Geometry: final body of the model. Coordinates: model frame, mm. A direction names the side the tool comes from. Round coordinates to 2 decimals unless told otherwise and drop trailing zeros. Write each loop counter-clockwise with the first axis right and the second up, starting at its lowest first coordinate (ties: lowest second). Pieces come first, ordered by that corner, then holes. Notation, with made-up numbers: (29.25, 31.5) -> (73.25, 31.5) arc R17 cw to (73.25, 57.5) -> close; hole circle Ø5 at (75.5, 72.25). An arc over 180 degrees is marked (long way). One line per item, written item: value. Start each with the question number.
from build123d import *

# Parameters (mm, degrees)
SKETCH1_R               = 10
BOSS_EXTRUDE1_DEPTH     = 35
SKETCH2_R               = 2.9
CUT_EXTRUDE1_DEPTH      = 12
CUT_EXTRUDE1_DRAFT      = -1
CUT_EXTRUDE2_DEPTH      = 38.749172176
CUT_EXTRUDE2_DEPTH_BACK = 38.749172176
SKETCH3_R               = 3
CUT_EXTRUDE3_REACH      = 39.749
CUT_EXTRUDE3_END_RADIUS = 3
SKETCH4_R               = 2.8


with BuildPart() as part:
    # Sketch1 → Boss-Extrude1 (new body)
    with BuildSketch(Plane.XY):
        Circle(SKETCH1_R)
    extrude(amount=BOSS_EXTRUDE1_DEPTH)


with BuildPart() as cut_extrude1_tool:
    # Sketch2 → Cut-Extrude1 (with draft: the straight prism first)
    with BuildSketch(Plane(origin=(0, 0, 12), x_dir=(-1, 0, 0), z_dir=(0, 0, -1))):
        Circle(SKETCH2_R)
    extrude(amount=CUT_EXTRUDE1_DEPTH)
    # Cut-Extrude1: the draft: its side faces are tilted about the plane it starts from
    cut_extrude1_sides = [cut_extrude1_tool.faces().sort_by_distance(p)[0] for p in [
        (2.9, 0, 6),
    ]]
    draft(cut_extrude1_sides, Plane(origin=(0, 0, 12), x_dir=(-1, 0, 0), z_dir=(0, 0, -1)), CUT_EXTRUDE1_DRAFT)


with BuildPart() as part_1:
    add(part.part)

    # Cut-Extrude1: cut by cut_extrude1_tool
    add(cut_extrude1_tool.part, mode=Mode.SUBTRACT)

    # Sketch3 → Cut-Extrude2 (cut, two sides: drawn at the far end of the back side and taken through both)
    with BuildSketch(Plane(origin=(0, 0, 0), x_dir=(1, 0, 0), z_dir=(0, 1, 0)).offset(-CUT_EXTRUDE2_DEPTH_BACK)):
        with Locations(Location((0, -25, 0), (0, 0, 270))):
            Circle(SKETCH3_R)
    extrude(amount=CUT_EXTRUDE2_DEPTH + CUT_EXTRUDE2_DEPTH_BACK, mode=Mode.SUBTRACT)

    # Cut-Extrude3: up to this cylinder (the profile starts outside it)
    cut_extrude3_end = Plane(origin=(0, 0, 25), z_dir=(0, 1, 0)) * Cylinder(CUT_EXTRUDE3_END_RADIUS, 86.498, mode=Mode.PRIVATE)
    # Sketch4 → Cut-Extrude3 (cut, up to the surface)
    with BuildSketch(Plane.XY.offset(35), mode=Mode.PRIVATE) as cut_extrude3_sk1:
        Circle(SKETCH4_R)
    cut_extrude3_tool1 = extrude(cut_extrude3_sk1.sketch, amount=-CUT_EXTRUDE3_REACH, mode=Mode.PRIVATE) - cut_extrude3_end
    add(cut_extrude3_tool1.solids().sort_by_distance((0, 0, 35))[0], mode=Mode.SUBTRACT)


solid = part_1.part
(1) Section query D-D (z = 32). Output: boundary loops of the cut face in (x, y), and give its area (3 significant figures).
(2) Section query B-B (x = 0). Count the separate pieces of the cut face and the enclosed holes in it, and give its area (3 significant figures).
(3) Pull-direction query (X, two-part tool) for faces 4 (the face through (-1.386, -2.664, 6.084)), 5 (the face through (9.54, 3, 17.26)), 6 (the face through (2.1, -2.1, 35)); classes: pulls with the +X half, pulls with the -X half, needs draft (parallel to the pull), parting line crosses it, or undercut.
(4) Pin query (flat end, axial travel): pin 1 (1.5 mm diameter, centred on y = -3.5, z = 6.5, fed in from +X); pin 2 (1.7 mm diameter, centred on x = 0, y = 0, fed in from -Z); pin 3 (9 mm diameter, centred on x = 0, y = 0, fed in from +Z); pin 4 (2 mm diameter, centred on y = 6.5, z = 8.5, fed in from -X). Return the tip coordinate at first contact, or that it passes through.
(5) Section query C-C (z = 21). Output: boundary loops of the cut face in (x, y).
(6) Line query: probe 1 along Y at (x, z) = (0, 29); probe 2 along X at (y, z) = (2, 29.5); probe 3 along X at (y, z) = (-2.75, 26.5). Output: solid intervals per line, ascending.
(7) Section query A-A (y = -8). Output: boundary loops of the cut face in (x, z), and give its area (3 significant figures).
(8) Set-up query: faces 1 (the face through (0, 0, 22)), 2 (the face through (0, 0, 12)), 3 (the face through (1.51, 2.36, 30.6)). Return all of +Z, -Z, +X, -X, +Y, -Y with unobstructed straight access to the full face (end or side cutting, diameter ignored); none if empty.
Results list:
1. outline: circle Ø20 at (0, 0); hole circle Ø5.6 at (0, 0)
1. area: 290 mm^2
2. separate pieces: 3
2. enclosed holes: 0
2. area: 469 mm^2
3. face 4: undercut
3. face 5: parting line crosses it
3. face 6: needs draft
4. pin 1: stops at x = 9.61
4. pin 2: stops at z = 12
4. pin 3: stops at z = 35
4. pin 4: stops at x = -8.35
5. outline: circle Ø20 at (0, 0)
6. probe 1: y = -10 to -2.8, 2.8 to 10
6. probe 2: x = -9.8 to -1.96, 1.96 to 9.8
6. probe 3: x = -9.61 to -2.6, 2.6 to 9.61
7. outline: (-6, 0) -> (6, 0) -> (6, 35) -> (-6, 35) -> close; hole circle Ø6 at (0, 25)
7. area: 392 mm^2
8. face 1: +Y, -Y
8. face 2: -Z
8. face 3: +Z
